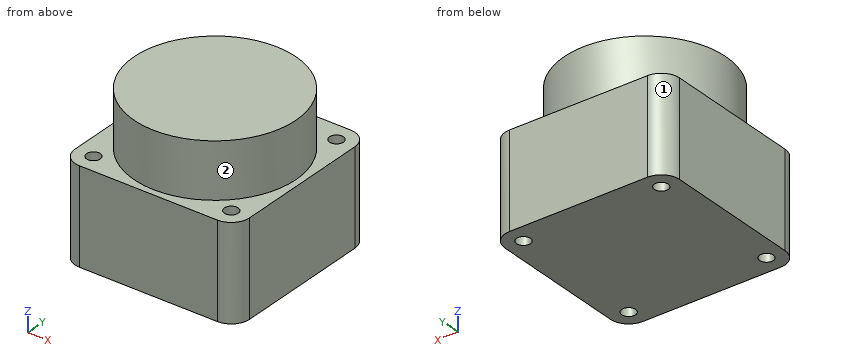
```python
from build123d import *

# Parameters (mm, degrees)
SKETCH_W     = 38
SKETCH_H     = 38
SKETCH_R     = 1.5
PAD_DEPTH    = 20.5
SKETCH001_R  = 17.6
PAD001_DEPTH = 12
FILLET_R     = 4


with BuildPart() as part:
    # Sketch → Pad (new body)
    with BuildSketch(Plane.XY):
        with Locations((29, 29)):
            Rectangle(SKETCH_W, SKETCH_H)
        with Locations((14, 14)):
            Circle(SKETCH_R, mode=Mode.SUBTRACT)
        with Locations((14, 44)):
            Circle(SKETCH_R, mode=Mode.SUBTRACT)
        with Locations((44, 44)):
            Circle(SKETCH_R, mode=Mode.SUBTRACT)
        with Locations((44, 14)):
            Circle(SKETCH_R, mode=Mode.SUBTRACT)
    extrude(amount=PAD_DEPTH)

    # Sketch001 (on Face10 of Pad) → Pad001 (join)
    with BuildSketch(Plane.XY.offset(20.5)):
        with Locations((29, 29)):
            Circle(SKETCH001_R)
    extrude(amount=PAD001_DEPTH)

    # Fillet
    fillet_edges = [part.edges().sort_by_distance(p)[0] for p in [
        (48, 10, 10.25),
        (48, 48, 10.25),
        (10, 48, 10.25),
        (10, 10, 10.25),
    ]]
    fillet(fillet_edges, radius=FILLET_R)


solid = part.part
```
The listing builds one solid part. Answer for the finished solid, in the listing's coordinates (mm). Face numbers are marked on the shaded views. A direction names the side the tool comes from. Coordinates: 2 decimals unless noted, no trailing zeros. Loops run counter-clockwise (first coordinate to the right, second up) from the corner with the lowest first, then second, coordinate; pieces in that order, holes last. Notation, with made-up numbers: (22, 31) -> (66, 31) arc R21 ccw to (66, 69) -> close; hole circle Ø4 at (28, 77). An arc over 180 degrees is marked (long way). Use one line per item in the form item = value. Start each with the question number.
Item 1: Consider L1, parallel to Y at x = 14, z = 16.75; L2, parallel to Y at x = 13, z = 11; L3, parallel to Z at x = 21.5, y = 12. Determine where each line is inside the solid, lowest interval first. Write a range as [from, to].
Item 2: The part is cut by section B-B on y = 29. Determine the outline of the cut face in (x, z), then the cut area to 3 significant figures.
Item 3: The part is cut by section C-C on x = 20.5. Determine the outline of the cut face in (y, z).
Item 4: The part is cut by section D-D on z = 26. Determine the outline of the cut face in (x, y), then the cut area to 3 significant figures.
Item 5: Flat-ended cylindrical pins translate along their axes: pin 1 Ø5 at (x, z) = (14, 28.5) entering from -Y; pin 2 Ø5 at (y, z) = (28, 26.5) entering from -X. Find the tip coordinate at first contact, or state that the pin passes through.
Item 6: A tool of negligible diameter and unlimited length cuts with its end or side. For the marked faces 1 and 2, from which of +Z, -Z, +X, -X, +Y, -Y can it reach the whole face along a straight path? Write none if from no direction.
Item 7: The part is cut by section A-A on z = 19.5. Determine the outline of the cut face in (x, y), then the cut area to 3 significant figures.
Answer key:
q1.L1 = [10, 12.5], [15.5, 42.5], [45.5, 48]
q1.L2 = [10.13, 12.88], [15.12, 42.88], [45.12, 47.87]
q1.L3 = [0, 20.5]
q2.outline = (10, 0) -> (48, 0) -> (48, 20.5) -> (46.6, 20.5) -> (46.6, 32.5) -> (11.4, 32.5) -> (11.4, 20.5) -> (10, 20.5) -> close
q2.area = 1,200 mm2
q3.outline = (10, 0) -> (48, 0) -> (48, 20.5) -> (44.41, 20.5) -> (44.41, 32.5) -> (13.59, 32.5) -> (13.59, 20.5) -> (10, 20.5) -> close
q4.outline = circle Ø35.2 at (29, 29)
q4.area = 973 mm2
q5.pin_1 = 16.61
q5.pin_2 = 11.4
q6.face_1 = +Z, -Z, -X, +Y
q6.face_2 = +Z
q7.outline = (10, 14) arc R4 ccw to (14, 10) -> (44, 10) arc R4 ccw to (48, 14) -> (48, 44) arc R4 ccw to (44, 48) -> (14, 48) arc R4 ccw to (10, 44) -> close; hole circle Ø3 at (14, 14); hole circle Ø3 at (14, 44); hole circle Ø3 at (44, 14); hole circle Ø3 at (44, 44)
q7.area = 1,400 mm2
